from build123d import *

# Parameters (mm, degrees)
F0_W     = 55
F0_H     = 90
F1_DEPTH = 3
F2_R     = 4.25
F3_DEPTH = 3
F4_R     = 5
F5_R     = 2.75
F6_DEPTH = 3


with BuildPart() as f1:
    # F0 (on Front) → F1 (new body)
    with BuildSketch(Plane.XZ):
        Rectangle(F0_W, F0_H)
    extrude(amount=F1_DEPTH)

    # F2 (on face) → F3 (cut, through all)
    with BuildSketch(Plane.XZ.offset(3)):
        with Locations((0, 27.5)):
            Circle(F2_R)
    extrude(amount=-F3_DEPTH, mode=Mode.SUBTRACT)

    # F4
    f4_edges = [f1.edges().sort_by_distance(p)[0] for p in [
        (-27.5, -1.5, 45),
        (27.5, -1.5, 45),
        (27.5, -1.5, -45),
        (-27.5, -1.5, -45),
    ]]
    fillet(f4_edges, radius=F4_R)

    # F5 (on face) → F6 (cut, through all)
    with BuildSketch(Plane.XZ.offset(3)):
        with Locations((0, -22.5)):
            Circle(F5_R)
    extrude(amount=-F6_DEPTH, mode=Mode.SUBTRACT)


solid = f1.part
Part model, mm, in its own coordinate system. Give positions to 0.01 mm unless a question says otherwise; leave off trailing zeros. Write each loop counter-clockwise with the first axis right and the second up, starting at its lowest first coordinate (ties: lowest second). Pieces come first, ordered by that corner, then holes.
1) Pin check, flat tips, straight feed: pin 1 (12 mm diameter, centred on x = -13.5, z = 4, fed in from +Y); pin 2 (3.5 mm diameter, centred on x = 0, z = -22.5, fed in from -Y). Stop position of each tip, or through.
Resolved:
pin 1: stops at y = 0
pin 2: passes through
2) Probe L1, parallel to Z at x = 0, y = -0.95; L2, parallel to X at y = -2.9, z = 29.5; L3, parallel to X at y = -0.5, z = 24. List the from-to ranges inside material, lowest first.
Resolved:
L1: z = -45 to -25.25, -19.75 to 23.25, 31.75 to 45
L2: x = -27.5 to -3.75, 3.75 to 27.5
L3: x = -27.5 to -2.41, 2.41 to 27.5
3) Cut at B-B on z = 27.5. Write the cut outline in (x, y).
Resolved:
outline: (-27.5, -3) - (-4.25, -3) - (-4.25, 0) - (-27.5, 0) - close; (4.25, -3) - (27.5, -3) - (27.5, 0) - (4.25, 0) - close
4) Cut at A-A on x = 0. Write the cut outline in (y, z).
Resolved:
outline: (-3, -45) - (0, -45) - (0, -25.25) - (-3, -25.25) - close; (-3, -19.75) - (0, -19.75) - (0, 23.25) - (-3, 23.25) - close; (-3, 31.75) - (0, 31.75) - (0, 45) - (-3, 45) - close
5) Cut at D-D on z = -22.5. Write the cut outline in (x, y).
Resolved:
outline: (-27.5, -3) - (-2.75, -3) - (-2.75, 0) - (-27.5, 0) - close; (2.75, -3) - (27.5, -3) - (27.5, 0) - (2.75, 0) - close
6) Cut at C-C on y = -1.85. Write the cut outline in (x, z).
Resolved:
outline: (-27.5, -40) arc R5 ccw to (-22.5, -45) - (22.5, -45) arc R5 ccw to (27.5, -40) - (27.5, 40) arc R5 ccw to (22.5, 45) - (-22.5, 45) arc R5 ccw to (-27.5, 40) - close; hole circle Ø8.5 at (0, 27.5); hole circle Ø5.5 at (0, -22.5)
7) Two-plate mould, pull along Z, no slides. Class faces 1 (the face through (2.285, -1.521, 31.084)), 2 (the face through (-0.358, -1.521, -19.773)), 3 (the face through (0, -1, 45)), 4 (the face through (0, -1, -45)): released by +Z, released by -Z, zero draft, split by the parting line, or undercut.
Resolved:
face 1: undercut
face 2: undercut
face 3: released by +Z
face 4: released by -Z
